Verification items for the finished model (mm, model axes). A direction names the side the tool comes from. Round coordinates to 2 decimals unless told otherwise and drop trailing zeros. Loops run counter-clockwise (first coordinate to the right, second up) from the corner with the lowest first, then second, coordinate; pieces in that order, holes last.
from build123d import *

# Parameters (mm, degrees)
SKETCH_1_W      = 10
SKETCH_1_H      = 10
EXTRUDE_1_DEPTH = 5
FILLET_2_R      = 2
SKETCH_2_R      = 2
EXTRUDE_2_DEPTH = 1


with BuildPart() as part:
    # 草图1 → 凸台-拉伸1 (new body)
    with BuildSketch(Plane(origin=(0, 0, 0), x_dir=(1, 0, 0), z_dir=(0, 1, 0))):
        Rectangle(SKETCH_1_W, SKETCH_1_H)
    extrude(amount=EXTRUDE_1_DEPTH)

    # 圆角2
    fillet_2_edges = [part.edges().sort_by_distance(p)[0] for p in [
        (5, 5, 0),
        (0, 5, 5),
        (-5, 5, 0),
        (0, 0, 5),
        (5, 0, 0),
        (0, 0, -5),
        (-5, 0, 0),
        (-5, 2.5, 5),
        (5, 2.5, 5),
        (5, 2.5, -5),
        (-5, 2.5, -5),
        (0, 5, -5),
    ]]
    fillet(fillet_2_edges, radius=FILLET_2_R)

    # 草图2 → 凸台-拉伸2 (add)
    with BuildSketch(Plane(origin=(0, 5, 0), x_dir=(1, 0, 0), z_dir=(0, 1, 0))):
        Circle(SKETCH_2_R)
    extrude(amount=EXTRUDE_2_DEPTH)


solid = part.part
1. Section check A-A (z = 2.25). Enter the section's corners in (x, y).
2. Scan lines: L1, parallel to Y at x = 2.25, z = 0.25; L2, parallel to X at y = 1.25, z = 1.5; L3, parallel to Y at x = -3.75, z = -3. Record each from-to range of solid material in increasing order.
3. Section check D-D (z = 0). Enter the section's corners in (x, y).
4. Section check C-C (y = 1.7). Enter the section's corners in (x, z), then the cut area to 3 significant figures.
5. Section check B-B (x = 0). Enter the section's corners in (y, z).
6. Tool access check on faces 1 (the face through (-1, 5, -2)), 2 (the face through (4.43, 2.51, -4.4)). Record the directions out of +Z, -Z, +X, -X, +Y, -Y that give a thin tool (end or side, any length) a straight path to the whole face; none if there is none.
7. Gauge pin test, flat ends, axial feed: P1, Ø2, axis at x = -2, y = 5.5, coming from the -Z side; P2, Ø1, axis at x = -3.5, y = 3.5, coming from the -Z side; P3, Ø4, axis at x = 1.5, z = 4, coming from the +Y side. Record the tip position at first contact, or that the pin passes through.
Taken from the geometry:
1. outline: (-5, 2) arc R2 ccw to (-3, 0) - (3, 0) arc R2 ccw to (5, 2) - (5, 3) arc R2 ccw to (3, 5) - (-3, 5) arc R2 ccw to (-5, 3) - close
2. L1: y = 0 to 5
2. L2: x = -4.85 to 4.85
2. L3: y = 0.15 to 4.85
3. outline: (-5, 2) arc R2 ccw to (-3, 0) - (3, 0) arc R2 ccw to (5, 2) - (5, 3) arc R2 ccw to (3, 5) - (2, 5) - (2, 6) - (-2, 6) - (-2, 5) - (-3, 5) arc R2 ccw to (-5, 3) - close
4. outline: (-4.98, -3) arc R1.98 ccw to (-3, -4.98) - (3, -4.98) arc R1.98 ccw to (4.98, -3) - (4.98, 3) arc R1.98 ccw to (3, 4.98) - (-3, 4.98) arc R1.98 ccw to (-4.98, 3) - close
4. area: 95.7 mm2
5. outline: (0, -3) arc R2 ccw to (2, -5) - (3, -5) arc R2 ccw to (5, -3) - (5, -2) - (6, -2) - (6, 2) - (5, 2) - (5, 3) arc R2 ccw to (3, 5) - (2, 5) arc R2 ccw to (0, 3) - close
6. face 1: +Y
6. face 2: -Z, +X, +Y, -Y
7. P1: stops at z = -4.32
7. P2: stops at z = -4.99
7. P3: stops at y = 5
